```python
from build123d import *

# Parameters (mm, degrees)
BOSS_EXTRUDE1_DEPTH = 1.5
BOSS_EXTRUDE2_DEPTH = 3
SKETCH3_W           = 3
SKETCH3_H           = 3
BOSS_EXTRUDE3_DEPTH = 1


with BuildPart() as part:
    # Sketch1 → Boss-Extrude1 (new body, symmetric)
    with BuildSketch(Plane.XY):
        with BuildLine():
            Line((-12.5, 2.5), (12.5, 2.5))
            ThreePointArc((12.5, 2.5), (15, 0), (12.5, -2.5))
            Line((12.5, -2.5), (-12.5, -2.5))
            ThreePointArc((-12.5, -2.5), (-15, 0), (-12.5, 2.5))
        make_face()
        with BuildLine():
            Line((-12.5, 1.65), (12.5, 1.65))
            ThreePointArc((12.5, 1.65), (14.15, 0), (12.5, -1.65))
            Line((12.5, -1.65), (-12.5, -1.65))
            ThreePointArc((-12.5, -1.65), (-14.15, 0), (-12.5, 1.65))
        make_face(mode=Mode.SUBTRACT)
    extrude(amount=BOSS_EXTRUDE1_DEPTH, both=True)

    # Sketch2 → Boss-Extrude2 (add)
    with BuildSketch(Plane.XY.offset(1.5)):
        with BuildLine():
            Line((-15, 0), (-15, -2.5))
            Line((-15, -2.5), (-12.5, -2.5))
            ThreePointArc((-12.5, -2.5), (-14.267766953, -1.767766953), (-15, 0))
        make_face()
        with BuildLine():
            Line((12.5, -2.5), (15, -2.5))
            Line((15, -2.5), (15, 0))
            ThreePointArc((15, 0), (14.267766953, -1.767766953), (12.5, -2.5))
        make_face()
    extrude(amount=-BOSS_EXTRUDE2_DEPTH)

    # Sketch3 → Boss-Extrude3 (add)
    with BuildSketch(Plane.XZ.offset(2.5)):
        with Locations((-12.5, 0)):
            Rectangle(SKETCH3_W, SKETCH3_H)
        with Locations((12.5, 0)):
            Rectangle(SKETCH3_W, SKETCH3_H)
    extrude(amount=BOSS_EXTRUDE3_DEPTH)


solid = part.part
```
The listing builds one solid part. Answer for the finished solid, in the listing's coordinates (mm). A direction names the side the tool comes from. Give positions to 0.01 mm unless a question says otherwise; leave off trailing zeros. Order: outer loops, then holes, each group sorted by start corner. A loop starts at its lowest first (then second) coordinate and runs counter-clockwise, first axis right, second up. Notation, with made-up numbers: M -39.75,-33.5 L -22.75,-33.5 A12 ccw -22.75,-13.5 Z; hole C 86,56.25 d6. An arc over 180 degrees is marked long. Put each result on its own line as item: value. Start each with the question number.
Item 1: The part is cut by section B-B, the plane z = 1.1. Determine the outline of the cut face in (x, y), and give its area (3 significant figures).
Item 2: Which of the six approach directions +Z, -Z, +X, -X, +Y, -Y give full straight-line access (tool end or side, diameter ignored) to faces 1 (the face through (11, -3, 0)), 2 (the face through (14.15, 0.04, 0.02)), 3 (the face through (-14.5, -2.5, 0)), 4 (the face through (14.5, -2.5, 0))?
Item 3: The part is cut by section A-A, the plane x = -10.5. Determine the outline of the cut face in (y, z), and give its area (3 significant figures).
Item 4: The part is cut by section C-C, the plane y = 1.15. Determine the outline of the cut face in (x, z).
Item 5: For a pull along Y with two mould halves and no side action, classify faces 5 (the face through (0, 2.5, 0)), 6 (the face through (-13, -3.5, 0)), 7 (the face through (-14, -3, 0)), 8 (the face through (0, 1.65, 0)) as +Y half, -Y half, draft (parallel to the pull), parting line (faces both ways), or undercut.
Item 6: Flat-ended cylindrical pins translate along their axes: P1, Ø0.9, axis at x = -3, z = 0.5, coming from the -Y side; P2, Ø3, axis at x = 0, y = 0, coming from the -Z side; P3, Ø0.5, axis at y = -3, z = 0.5, coming from the +X side; P4, Ø0.8, axis at y = -3, z = 0.5, coming from the -X side. Find the tip coordinate at first contact, or state that the pin passes through.
Item 7: Find the intervals of material crossed by line 1 along Y through (x, z) = (-4, -0.25); line 2 along Y through (x, z) = (-12, -0.3); line 3 along X through (y, z) = (-0.1, -0.45), in increasing order.
Answer key:
1. outline: M -15,-2.5 L -14,-2.5 L -14,-3.5 L -11,-3.5 L -11,-2.5 L 11,-2.5 L 11,-3.5 L 14,-3.5 L 14,-2.5 L 15,-2.5 L 15,0 A2.5 ccw 12.5,2.5 L -12.5,2.5 A2.5 ccw -15,0 Z; hole M -12.5,-1.65 L 12.5,-1.65 A1.65 ccw 12.5,1.65 L -12.5,1.65 A1.65 ccw Z
1. area: 62.3 mm²
2. face 1: +Z, -Z, -Y
2. face 2: +Z, -Z
2. face 3: +Z, -Z, -X, -Y
2. face 4: +Z, -Z, +X, -Y
3. outline: M -2.5,-1.5 L -1.65,-1.5 L -1.65,1.5 L -2.5,1.5 Z; M 1.65,-1.5 L 2.5,-1.5 L 2.5,1.5 L 1.65,1.5 Z
3. area: 5.10 mm²
4. outline: M -14.72,-1.5 L -13.68,-1.5 L -13.68,1.5 L -14.72,1.5 Z; M 13.68,-1.5 L 14.72,-1.5 L 14.72,1.5 L 13.68,1.5 Z
5. face 5: +Y half
5. face 6: -Y half
5. face 7: draft
5. face 8: undercut
6. P1: stops at y = -2.5
6. P2: passes through
6. P3: stops at x = 14
6. P4: stops at x = -14
7. line 1: y = -2.5 to -1.65, 1.65 to 2.5
7. line 2: y = -3.5 to -1.65, 1.65 to 2.5
7. line 3: x = -15 to -14.15, 14.15 to 15
